Can you work these out from the model? Positions are in its coordinate system, mm. Round coordinates to 2 decimals unless told otherwise and drop trailing zeros. Loops run counter-clockwise (first coordinate to the right, second up) from the corner with the lowest first, then second, coordinate; pieces in that order, holes last. Notation, with made-up numbers: (12.5, 2) - (50.5, 2) arc R20 ccw to (50.5, 38) - close; hole circle Ø7 at (24, -5). An arc over 180 degrees is marked (long way). Answer as CSV lines item,"result".
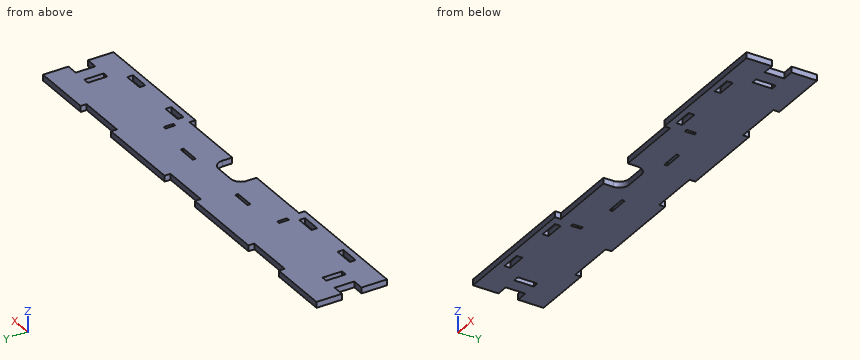
```python
from build123d import *

# Parameters (mm, degrees)
SKETCH_1_W      = 20
SKETCH_1_H      = 6
SKETCH_1_W_2    = 6
SKETCH_1_H_2    = 20
SKETCH_1_W_3    = 3
SKETCH_1_H_3    = 10
SKETCH_1_H_4    = 3
EXTRUDE_1_DEPTH = 6
FILLET_1_R      = 10
FILLET_2_R      = 10


with BuildPart() as part:
    # Эскиз1 → Бобышка-Вытянуть1 (new body)
    with BuildSketch(Plane.XY):
        Polygon((0, 60), (0, 66), (62, 66), (62, 60), (112, 60), (112, 66), (200, 66), (200, 60), (250, 60), (250, 66), (338, 66), (338, 60), (388, 60), (388, 66), (450, 66), (450, 60), (450, 40), (438, 40), (438, 20), (450, 20), (450, 0), (450, -6), (315, -6), (315, 0), (245, 0), (245, 20), (205, 20), (205, 0), (135, 0), (135, -6), (0, -6), (0, 0), (0, 20), (12, 20), (12, 40), (0, 40), align=None)
        with Locations((115, 3)):
            Rectangle(SKETCH_1_W, SKETCH_1_H, mode=Mode.SUBTRACT)
        with Locations((335, 3)):
            Rectangle(SKETCH_1_W, SKETCH_1_H, mode=Mode.SUBTRACT)
        with Locations((29, 30)):
            Rectangle(SKETCH_1_W_2, SKETCH_1_H_2, mode=Mode.SUBTRACT)
        with Locations((421, 30)):
            Rectangle(SKETCH_1_W_2, SKETCH_1_H_2, mode=Mode.SUBTRACT)
        with Locations((398, 3)):
            Rectangle(SKETCH_1_W, SKETCH_1_H, mode=Mode.SUBTRACT)
        with Locations((52, 3)):
            Rectangle(SKETCH_1_W, SKETCH_1_H, mode=Mode.SUBTRACT)
        with Locations((318.5, 18.5)):
            Rectangle(SKETCH_1_W_3, SKETCH_1_H_3, mode=Mode.SUBTRACT)
        with Locations((131.5, 18.5)):
            Rectangle(SKETCH_1_W_3, SKETCH_1_H_3, mode=Mode.SUBTRACT)
        with Locations((180, 29.5)):
            Rectangle(SKETCH_1_W, SKETCH_1_H_4, mode=Mode.SUBTRACT)
        with Locations((270, 29.5)):
            Rectangle(SKETCH_1_W, SKETCH_1_H_4, mode=Mode.SUBTRACT)
    extrude(amount=EXTRUDE_1_DEPTH)

    # Скругление1
    fillet_1_edges = [part.edges().sort_by_distance(p)[0] for p in [
        (205, 20, 3),
    ]]
    fillet(fillet_1_edges, radius=FILLET_1_R)

    # Скругление2
    fillet_2_edges = [part.edges().sort_by_distance(p)[0] for p in [
        (245, 20, 3),
    ]]
    fillet(fillet_2_edges, radius=FILLET_2_R)


solid = part.part
```
Q1. Imagine slicing it at C-C (z = 4.25). Count the separate pieces of the cut face and the enclosed holes in it, then the cut area to 3 significant figures.
Checks:
separate pieces,"1"
enclosed holes,"10"
area,"28,300 mm²"
Q2. Imagine slicing it at A-A (x = 272). Write out the boundary of the cut face in (y, z).
Checks:
outline,"(0, 0) - (28, 0) - (28, 6) - (0, 6) - close; (31, 0) - (66, 0) - (66, 6) - (31, 6) - close"
Q3. Imagine slicing it at D-D (x = 96.5). Write out the boundary of the cut face in (y, z), then the cut area to 3 significant figures.
Checks:
outline,"(-6, 0) - (60, 0) - (60, 6) - (-6, 6) - close"
area,"396 mm²"
Q4. I'm going to push flat-ended pins straight in: pin 1 Ø2 at (y, z) = (33.5, 2) entering from +X; pin 2 Ø3 at (x, z) = (351, 4) entering from +Y; pin 3 Ø3 at (y, z) = (34, 3) entering from -X. Where does each tip first touch, or does it pass through?
Checks:
pin 1,"x = 438"
pin 2,"y = 60"
pin 3,"x = 12"
Q5. Imagine slicing it at B-B (x = 329.5). Write out the boundary of the cut face in (y, z).
Checks:
outline,"(-6, 0) - (0, 0) - (0, 6) - (-6, 6) - close; (6, 0) - (66, 0) - (66, 6) - (6, 6) - close"
Q6. If I drill on line 1 along X through (y, z) = (24, 3.1); line 2 along Y through (x, z) = (279, 1.3); line 3 along X through (y, z) = (9.5, 0.6), over which ranges is the centre line in solid material (lowest first)? Write a range as [from, to].
Checks:
line 1,"[12, 26], [32, 418], [424, 438]"
line 2,"[0, 28], [31, 66]"
line 3,"[0, 205], [245, 450]"
